Model file for the job. Use its own axes, mm. A direction names the side the tool comes from. Give positions to 0.01 mm unless a question says otherwise; leave off trailing zeros. Order: outer loops, then holes, each group sorted by start corner. A loop starts at its lowest first (then second) coordinate and runs counter-clockwise, first axis right, second up. Notation, with made-up numbers: (23, -16) -> (64, -16) arc R30 cw to (64, 8) -> close; hole circle Ø2 at (29, 68.25). An arc over 180 degrees is marked (long way). Use CSV: the item, a comma, the result in double quotes. Start each with the question number.
1. Pull direction X, two halves, no side cores. Call faces 5 (the flat face through (4.91, 23, 3)), 6 (the flat face through (-2, -72.494, 6)), 7 (the flat face through (2.91, -11, 5)), 8 (the conical face through (-6.567, 207.533, 1.424)): released by +X, released by -X, zero draft, split by the parting line, or undercut.
2. 3-axis set-ups, long thin cutter, end or side, ignore diameter. For faces 1 (the flat face through (-13, -42.494, 4)), 2 (the flat face through (-9.09, 22, 3)), 3 (the flat face through (9, -42.494, 4)), 4 (the flat face through (-2, -42.494, 9)): which of +Z, -Z, +X, -X, +Y, -Y reach the whole face in a straight line?
3. Cut at C-C on z = 2.5. List the corners of the cut face in (x, y), then the cut area to 3 significant figures.
4. Wall check: line 1 (X direction, y = 57.5, z = 5.5); line 2 (X direction, y = 33, z = 2); line 3 (Z direction, x = -11, y = 73.5). Give the ranges that are in metal, low to high. Write a range as from..to.
5. Cut at B-B on y = 92. List the corners of the cut face in (x, z).
6. Drop flat-ended pins along their axis: pin 1 (17 mm diameter, centred on x = 2, y = 81, fed in from +Z); pin 2 (1.8 mm diameter, centred on y = 42, z = 2.5, fed in from -X); pin 3 (3 mm diameter, centred on y = 174, z = 2, fed in from +X); pin 4 (2.5 mm diameter, centred on y = -59, z = 6, fed in from +X). Give the stop position or say it passes through.
7. Cut at A-A on y = -12.5. List the corners of the cut face in (x, z).
```python
from build123d import *

# Parameters (mm, degrees)
F1_DEPTH    = 6
F2_T1_DEPTH = 242.8543856465
F3_W        = 10
F3_H        = 30
F4_DEPTH    = 6
F5_R        = 1.5
F6_DEPTH    = 10
F7_SIZE     = 5


# Not quite as in the source:
# - a fillet or chamfer that OpenCascade refuses, or shapes differently, is made with other operations: its cross-section is extruded or revolved along the edge and cut away or added


with BuildPart() as f1:
    # F0 (on Top) → F1 (new body)
    with BuildSketch(Plane.XY):
        Polygon((14.9102990106, 227.5062542017), (-19.0897009894, 227.5062542017), (-19.0897009894, -42.4937457983), (-9.0897009894, -42.4937457983), (-9.0897009894, 87.5062542017), (-7.0897009894, 87.5062542017), (-7.0897009894, -72.4937457983), (2.9102990106, -72.4937457983), (2.9102990106, 87.5062542017), (4.9102990106, 87.5062542017), (4.9102990106, -42.4937457983), (14.9102990106, -42.4937457983), align=None)
    extrude(amount=F1_DEPTH)

    # F2: fillet of radius 50 on 1 edges, made by hand

    # F2_s2 → F2_t1 (cut)
    with BuildSketch(Plane.XY.offset(-118.4271928233)):
        with BuildLine():
            ThreePointArc((14.9102990106, 227.5062542017), (-9.7098930126, 209.2901365467), (-19.0897009894, 180.1353770724))
            Line((-19.0897009894, 180.1353770724), (-19.0897009894, 227.5062542017))
            Line((-19.0897009894, 227.5062542017), (14.9102990106, 227.5062542017))
        make_face()
    extrude(amount=F2_T1_DEPTH, mode=Mode.SUBTRACT)

    # F3 (on face) → F4 (join)
    with BuildSketch(Plane.XY.offset(6)):
        with Locations((-2.0897009894, -57.4937457983)):
            Rectangle(F3_W, F3_H)
    extrude(amount=F4_DEPTH)

    # F5 (on face) → F6 (cut, through all)
    with BuildSketch(Plane(origin=(-7.0897009894, 0, 0), x_dir=(0, -1, 0), z_dir=(-1, 0, 0))):
        with Locations((59.0019002557, 6)):
            Circle(F5_R)
    extrude(amount=-F6_DEPTH, mode=Mode.SUBTRACT)

    # F7
    f7_edges = [f1.edges().sort_by_distance(p)[0] for p in [
        (14.910299, 92.506254, 0),
        (-19.089701, 68.820816, 0),
        (-9.709893, 209.290137, 0),
    ]]
    chamfer(f7_edges, length=F7_SIZE)


solid = f1.part
```
Verdict:
1,face 5,"undercut"
1,face 6,"zero draft"
1,face 7,"undercut"
1,face 8,"released by -X"
2,face 1,"+Z, -Z, -X, -Y"
2,face 2,"+Z, -Z, -Y"
2,face 3,"+Z, -Z, +X, -Y"
2,face 4,"+Z, +X, -X, +Y"
3,outline,"(-16.59, -42.49) -> (-9.09, -42.49) -> (-9.09, 87.51) -> (-7.09, 87.51) -> (-7.09, -72.49) -> (2.91, -72.49) -> (2.91, 87.51) -> (4.91, 87.51) -> (4.91, -42.49) -> (12.41, -42.49) -> (12.41, 223.88) arc R47.5 ccw to (-16.59, 180.14) -> close"
3,area,"7,150 mm^2"
4,line 1,"-19.09..-9.09, -7.09..2.91, 4.91..14.91"
4,line 2,"-16.09..-9.09, -7.09..2.91, 4.91..11.91"
4,line 3,"0..6"
5,outline,"(-19.09, 5) -> (-14.09, 0) -> (9.91, 0) -> (14.91, 5) -> (14.91, 6) -> (-19.09, 6) -> close"
6,pin 1,"z = 6"
6,pin 2,"x = -17.49"
6,pin 3,"x = 13.41"
6,pin 4,"through"
7,outline,"(-19.09, 5) -> (-14.09, 0) -> (-9.09, 0) -> (-9.09, 6) -> (-19.09, 6) -> close; (-7.09, 0) -> (2.91, 0) -> (2.91, 6) -> (-7.09, 6) -> close; (4.91, 0) -> (9.91, 0) -> (14.91, 5) -> (14.91, 6) -> (4.91, 6) -> close"
